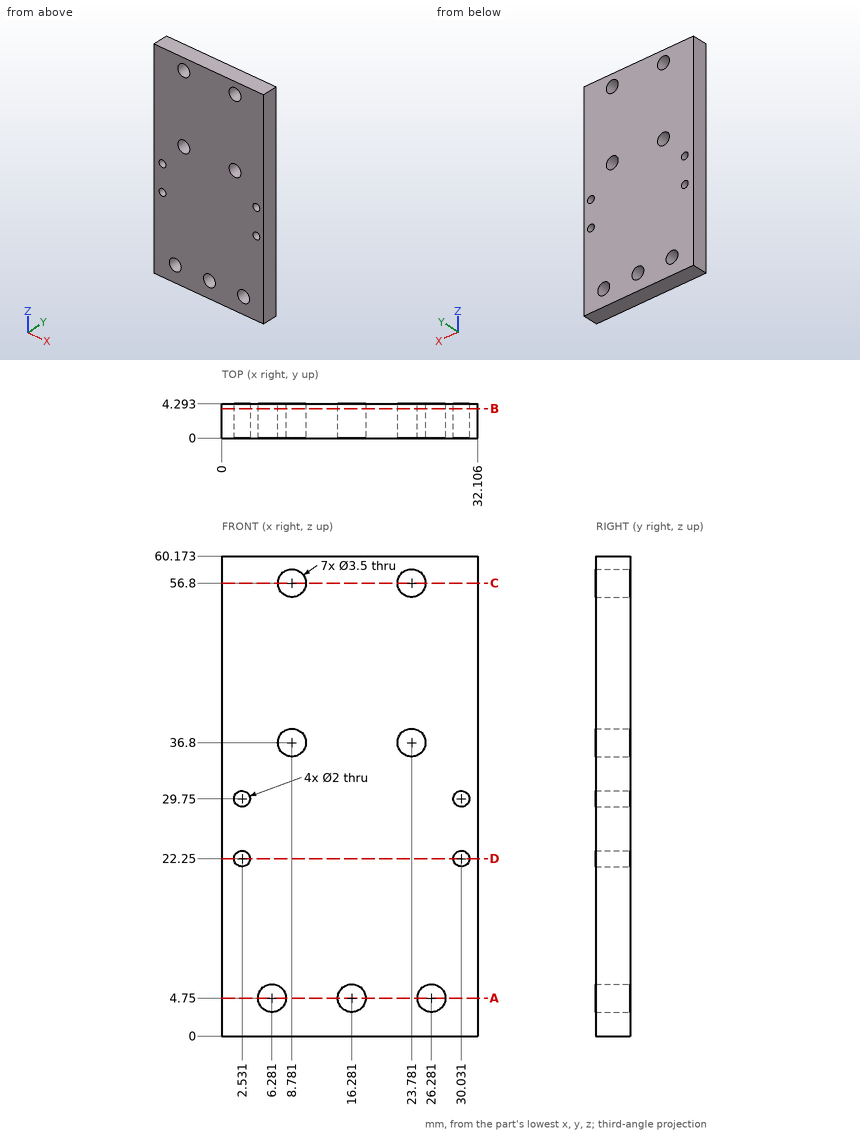
Drawing for the job (mm, zero at the part's lowest x, y, z). Coordinates: 2 decimals unless noted, no trailing zeros. Order: outer loops, then holes, each group sorted by start corner. A loop starts at its lowest first (then second) coordinate and runs counter-clockwise, first axis right, second up. Notation, with made-up numbers: (-17, -22.5) -> (0, -22.5) arc R20 cw to (0, 9.5) -> close; hole circle Ø9 at (52, 72.25). An arc over 180 degrees is marked (long way). One line per item, written item: value.
(1) Slice it at B-B, the plane y = 3.7. Count the separate pieces of the cut face and the enclosed holes in it, plus the area to 3 significant figures.
Checked values:
separate pieces: 1
enclosed holes: 11
area: 1,850 mm2
(2) Slice it at D-D, the plane z = 22.25. List the corners of the cut face in (x, y) (1 decimal), plus the area to 3 significant figures.
Checked values:
outline: (0, 0) -> (1.5, 0) -> (1.5, 4.3) -> (0, 4.3) -> close; (3.5, 0) -> (29, 0) -> (29, 4.3) -> (3.5, 4.3) -> close; (31, 0) -> (32.1, 0) -> (32.1, 4.3) -> (31, 4.3) -> close
area: 121 mm2
(3) Slice it at A-A, the plane z = 4.75. List the corners of the cut face in (x, y) (1 decimal).
Checked values:
outline: (0, 0) -> (4.5, 0) -> (4.5, 4.3) -> (0, 4.3) -> close; (8, 0) -> (14.5, 0) -> (14.5, 4.3) -> (8, 4.3) -> close; (18, 0) -> (24.5, 0) -> (24.5, 4.3) -> (18, 4.3) -> close; (28, 0) -> (32.1, 0) -> (32.1, 4.3) -> (28, 4.3) -> close
(4) Probe line 1 (Z direction, x = 2.5, y = 2.05); line 2 (X direction, y = 3.1, z = 23) (1 decimal); line 3 (Z direction, x = 8.5, y = 1.7). List the from-to ranges inside material, lowest first. Write a range as [from, to].
Checked values:
line 1: [0, 21.25], [23.25, 28.75], [30.75, 60.17]
line 2: [0, 1.9], [3.2, 29.4], [30.7, 32.1]
line 3: [0, 35.07], [38.53, 55.07], [58.53, 60.17]
(5) Slice it at C-C, the plane z = 56.8. List the corners of the cut face in (x, y) (1 decimal), plus the area to 3 significant figures.
Checked values:
outline: (0, 0) -> (7, 0) -> (7, 4.3) -> (0, 4.3) -> close; (10.5, 0) -> (22, 0) -> (22, 4.3) -> (10.5, 4.3) -> close; (25.5, 0) -> (32.1, 0) -> (32.1, 4.3) -> (25.5, 4.3) -> close
area: 108 mm2
